from build123d import *

# Parameters (mm, degrees)
SKETCH1_R           = 73.025
SKETCH1_R_2         = 3.3
BOSS_EXTRUDE1_DEPTH = 4.7625


with BuildPart() as part:
    # Sketch1 → Boss-Extrude1 (new body, symmetric)
    with BuildSketch(Plane(origin=(0, 0, 0), x_dir=(1, 0, 0), z_dir=(0, 1, 0))):
        Circle(SKETCH1_R)
        Circle(SKETCH1_R_2, mode=Mode.SUBTRACT)
        with Locations((0, -57.15)):
            Circle(SKETCH1_R_2, mode=Mode.SUBTRACT)
        with Locations((-49.493351826, 28.575)):
            Circle(SKETCH1_R_2, mode=Mode.SUBTRACT)
        with Locations((49.493351826, 28.575)):
            Circle(SKETCH1_R_2, mode=Mode.SUBTRACT)
        with Locations((24.746675913, -14.2875)):
            Circle(SKETCH1_R_2, mode=Mode.SUBTRACT)
        with Locations((-24.746675913, -14.2875)):
            Circle(SKETCH1_R_2, mode=Mode.SUBTRACT)
        with Locations((0, 28.575)):
            Circle(SKETCH1_R_2, mode=Mode.SUBTRACT)
    extrude(amount=BOSS_EXTRUDE1_DEPTH, both=True)


solid = part.part
CAD build for the part. Positions are in the model's coordinates, mm. Round coordinates to 2 decimals unless told otherwise and drop trailing zeros. Write each loop counter-clockwise with the first axis right and the second up, starting at its lowest first coordinate (ties: lowest second). Pieces come first, ordered by that corner, then holes. Notation, with made-up numbers: (17.25, 74) -> (29.25, 74) arc R26 ccw to (29.25, 98) -> close; hole circle Ø1 at (73.5, 60). An arc over 180 degrees is marked (long way). Answer as a JSON object with one key per item and string values.
(1) Band-saw the part on D-D, the plane z = 57.15. List the corners of the cut face in (x, y), then the cut area to 3 significant figures.
Reported:
{"outline": "(-45.46, -4.76) -> (-3.3, -4.76) -> (-3.3, 4.76) -> (-45.46, 4.76) -> close; (3.3, -4.76) -> (45.46, -4.76) -> (45.46, 4.76) -> (3.3, 4.76) -> close", "area": "803 mm^2"}
(2) Probe probe 1 along Z at (x, y) = (0, -1.75) (3 decimals); probe 2 along Z at (x, y) = (-0.5, -1); probe 3 along X at (y, z) = (-0.75, -29.5). List the from-to ranges inside material, lowest first. Write a range as [from, to].
Reported:
{"probe 1": "z = [-73.025, -31.875], [-25.275, -3.3], [3.3, 53.85], [60.45, 73.025]", "probe 2": "z = [-73.02, -31.84], [-25.31, -3.26], [3.26, 53.89], [60.41, 73.02]", "probe 3": "x = [-66.8, -52.66], [-46.33, -3.17], [3.17, 46.33], [52.66, 66.8]"}
(3) Band-saw the part on B-B, the plane x = 0. Count the separate pieces of the cut face and the enclosed holes in it, then the cut area to 3 significant figures.
Reported:
{"separate pieces": "4", "enclosed holes": "0", "area": "1,200 mm^2"}
(4) Band-saw the part on A-A, the plane z = 0. List the corners of the cut face in (x, y) (1 decimal).
Reported:
{"outline": "(-73, -4.8) -> (-3.3, -4.8) -> (-3.3, 4.8) -> (-73, 4.8) -> close; (3.3, -4.8) -> (73, -4.8) -> (73, 4.8) -> (3.3, 4.8) -> close"}
(5) Two-plate mould, pull along X, no slides. Class faces 1 (the face through (69.653, 0.067, -21.935)), 2 (the face through (-1, 4.762, 15)), 3 (the face through (46.87, -0.07, -26.57)): +X half, -X half, draft (parallel to the pull), parting line (faces both ways), or undercut.
Reported:
{"face 1": "parting line", "face 2": "draft", "face 3": "undercut"}
(6) Pin check, flat tips, straight feed: P1, Ø2, axis at y = -1.5, z = 16.5, coming from the -X side; P2, Ø5, axis at y = 3.5, z = 35, coming from the -X side; P3, Ø5, axis at y = 2, z = 35, coming from the +X side; P4, Ø4, axis at x = 49.49, z = -28.58, coming from the -Y side. Stop position of each tip, or through.
Reported:
{"P1": "stops at x = -71.36", "P2": "stops at x = -65.39", "P3": "stops at x = 65.39", "P4": "passes through"}
